Part model, mm, in its own coordinate system. A direction names the side the tool comes from. Round coordinates to 2 decimals unless told otherwise and drop trailing zeros. Loops run counter-clockwise (first coordinate to the right, second up) from the corner with the lowest first, then second, coordinate; pieces in that order, holes last.
1) 3-axis set-ups, long thin cutter, end or side, ignore diameter. For faces 1 (the flat face through (158.88, 67.338, 0.986)), 2 (the flat face through (26.209, 80.925, 0.986)): which of +Z, -Z, +X, -X, +Y, -Y reach the whole face in a straight line?
2) Mould opens along Y. For faces 3 (the flat face through (164.897, 26.653, 0.986)), 4 (the flat face through (89, 31, 2)), 5 (the flat face through (147.73, -10.78, 0.99)) say: +Y half, -Y half, draft (parallel to the pull), parting line (faces both ways), or undercut.
3) Probe line 1 (Y direction, x = 152.5, z = 0.4); line 2 (X direction, y = 79, z = 0.75); line 3 (X direction, y = 83, z = 1.35). List the from-to ranges inside material, lowest first.
4) Band-saw the part on A-A, the plane x = 168.5. Write the cut outline in (y, z), then the cut area to 3 significant figures.
5) Drop flat-ended pins along their axis: P1, Ø0.6, axis at x = 39.5, z = 1, coming from the +Y side; P2, Ø0.6, axis at y = 67, z = 1, coming from the -X side; P3, Ø0.6, axis at y = 53, z = 0.5, coming from the -X side. Give the stop position or say it passes through.
6) Band-saw the part on B-B, the plane y = -22.5. Write the cut outline in (x, z).
from build123d import *

# Parameters (mm, degrees)
AUFSATZ_LINEAR_AUSTRAGEN1_DEPTH = 2


with BuildPart() as part:
    # Skizze1 → Aufsatz-Linear austragen1 (new body)
    with BuildSketch(Plane.XY):
        Polygon((126.215995869, 93.72314004), (130.025876451, 93.72314004), (135.595633387, 97.38954443), (138.718293672, 95.556342235), (142.844671433, 96.629977996), (147.286818563, 95.556342235), (147.286818563, 93.72314004), (157.138174255, 91.342136563), (158.946705069, 92.532638301), (161.425092467, 90.311861568), (165.521072329, 87.907258253), (165.521072329, 84.158745075), (157.138174255, 79.801706236), (154.161759315, 79.027277499), (153.074965654, 77.17604286), (153.074965654, 76.08832996), (157.138174255, 75.10628098), (158.946705069, 73.485734023), (162.549971035, 70.257001813), (155.106569955, 64.335109931), (157.138174255, 50.240352889), (140.181002279, 42.752564778), (138.718293672, 42.752564778), (138.718293672, 29.895134459), (191.818980244, 23.319015351), (191.818980244, 12.135974598), (102.392093357, -34.343943925), (-17.273133713, -5.421699037), (20.56292279, 14.243715747), (20.56292279, 34.449415172), (17.079292064, 41.151884986), (18.821107427, 48.358612255), (25.556462177, 51.859335035), (34.70239759, 51.859335035), (34.70239759, 55.062538542), (17.950199746, 55.062538542), (17.950199746, 76.63218641), (34.70239759, 85.339196326), (41.469675345, 85.339196326), (51.303413636, 86.75662161), (62.052077393, 84.158745075), (62.052077393, 80.985691368), (73.7183454, 80.985691368), (73.7183454, 76.63218641), (83.622998605, 74.238301298), (83.622998605, 90.311861568), (93.594862899, 90.311861568), (96.253356842, 111.778603776), (99.649825979, 125.83142893), (105.714042553, 130.656056075), (123.966404927, 130.656056075), (126.215995869, 115.048962824), (128.761406921, 97.38954443), align=None)
    extrude(amount=AUFSATZ_LINEAR_AUSTRAGEN1_DEPTH)


solid = part.part
Reported:
1. face 1: +Z, -Z, +X
1. face 2: +Z, -Z, -X, +Y
2. face 3: undercut
2. face 4: draft
2. face 5: -Y half
3. line 1: y = -8.3 to 28.19, 48.19 to 92.46
3. line 2: x = 22.51 to 73.72, 83.62 to 154.15
3. line 3: x = 30.2 to 62.05, 83.62 to 163.29
4. outline: (0.02, 0) - (26.21, 0) - (26.21, 2) - (0.02, 2) - close
4. area: 52.4 mm2
5. P1: stops at y = 85.34
5. P2: stops at x = 17.95
5. P3: stops at x = 34.7
6. outline: (53.39, 0) - (125.18, 0) - (125.18, 2) - (53.39, 2) - close
